Design review of the part built by this model. Coordinates are the model's own, in mm. A direction names the side the tool comes from. Round coordinates to 2 decimals unless told otherwise and drop trailing zeros. Order: outer loops, then holes, each group sorted by start corner. A loop starts at its lowest first (then second) coordinate and runs counter-clockwise, first axis right, second up. Notation, with made-up numbers: (-19.5, 29) - (39.5, 29) arc R28 cw to (39.5, 53) - close; hole circle Ø1 at (2, 22). An arc over 180 degrees is marked (long way). Use CSV: the item, a comma, the result in double quotes.
from build123d import *

# Parameters (mm, degrees)
BOX017_W                     = 10
BOX017_H                     = 10
BOX017_DEPTH                 = 10
BOX018_W                     = 10
BOX018_H                     = 10
BOX018_DEPTH                 = 10
BOX019_W                     = 10
BOX019_H                     = 10
BOX019_DEPTH                 = 10
BOX021_W                     = 10
BOX021_H                     = 10
BOX021_DEPTH                 = 10
BOX020_W                     = 10
BOX020_H                     = 10
BOX020_DEPTH                 = 10
FUSION002004_PLACEMENT_ANGLE = 180


with BuildPart() as cubo017:
    # Box017 → Box017 (new body)
    with BuildSketch(Plane(origin=(30, 0, 0), x_dir=(1, 0, 0), z_dir=(0, 0, 1))):
        with Locations((5, 5)):
            Rectangle(BOX017_W, BOX017_H)
    extrude(amount=BOX017_DEPTH)


with BuildPart() as cubo018:
    # Box018 → Box018 (new body)
    with BuildSketch(Plane(origin=(10, 0, 0), x_dir=(1, 0, 0), z_dir=(0, 0, 1))):
        with Locations((5, 5)):
            Rectangle(BOX018_W, BOX018_H)
    extrude(amount=BOX018_DEPTH)


with BuildPart() as cubo019:
    # Box019 → Box019 (new body)
    with BuildSketch(Plane(origin=(20, 0, 0), x_dir=(1, 0, 0), z_dir=(0, 0, 1))):
        with Locations((5, 5)):
            Rectangle(BOX019_W, BOX019_H)
    extrude(amount=BOX019_DEPTH)


with BuildPart() as cubo021:
    # Box021 → Box021 (new body)
    with BuildSketch(Plane(origin=(0, 10, 0), x_dir=(1, 0, 0), z_dir=(0, 0, 1))):
        with Locations((5, 5)):
            Rectangle(BOX021_W, BOX021_H)
    extrude(amount=BOX021_DEPTH)


with BuildPart() as fusion002004:
    # Box020 → Box020 (new body)
    with BuildSketch(Plane.XY):
        with Locations((5, 5)):
            Rectangle(BOX020_W, BOX020_H)
    extrude(amount=BOX020_DEPTH)

    # Fusion002004: union Cubo017, Cubo018, Cubo019, Cubo021
    add(cubo017.part)
    add(cubo018.part)
    add(cubo019.part)
    add(cubo021.part)


with BuildPart() as fusion002004_1:
    # Fusion002004 placement: moved
    add(fusion002004.part.moved(Location((40, 0, 0))).rotate(Axis((40, 0, 0), (0, 0, 1)), FUSION002004_PLACEMENT_ANGLE))


solid = fusion002004_1.part
1) To check wall thickness, follow L1, parallel to X at y = -10.75, z = 6.25; L2, parallel to Y at x = 6, z = 6.25. State the ranges of each line that lie inside material, in increasing order. Write a range as from..to.
Data:
L1,"x = 30..40"
L2,"y = -10..0"
2) For faces 1 (the face through (30, -15, 5)), 2 (the face through (40, -10, 5)), list the 3-axis set-ups (+Z, -Z, +X, -X, +Y, -Y) from which the entire face can be reached by the end or side of a thin tool; tool diameter is ignored.
Data:
face 1,"+Z, -Z, -X, -Y"
face 2,"+Z, -Z, +X, +Y, -Y"
3) Insertion check: pin 1 Ø1.5 at (x, z) = (20, 7) entering from -Y; pin 2 Ø3 at (y, z) = (-17, 7.5) entering from -X. Each pin has a flat end and moves straight along its axis. Give the tip position at first contact, or say it passes through.
Data:
pin 1,"stops at y = -10"
pin 2,"stops at x = 30"
4) We need section C-C (x = 29). Give the boundary of the cut face in (y, z), then the cut area to 3 significant figures.
Data:
outline,"(-10, 0) - (0, 0) - (0, 10) - (-10, 10) - close"
area,"100 mm2"
5) We need section A-A (z = 6.5). Give the boundary of the cut face in (x, y).
Data:
outline,"(0, -10) - (30, -10) - (30, -20) - (40, -20) - (40, 0) - (0, 0) - close"
6) We need section B-B (y = -11). Give the boundary of the cut face in (x, z), then the cut area to 3 significant figures.
Data:
outline,"(30, 0) - (40, 0) - (40, 10) - (30, 10) - close"
area,"100 mm2"
